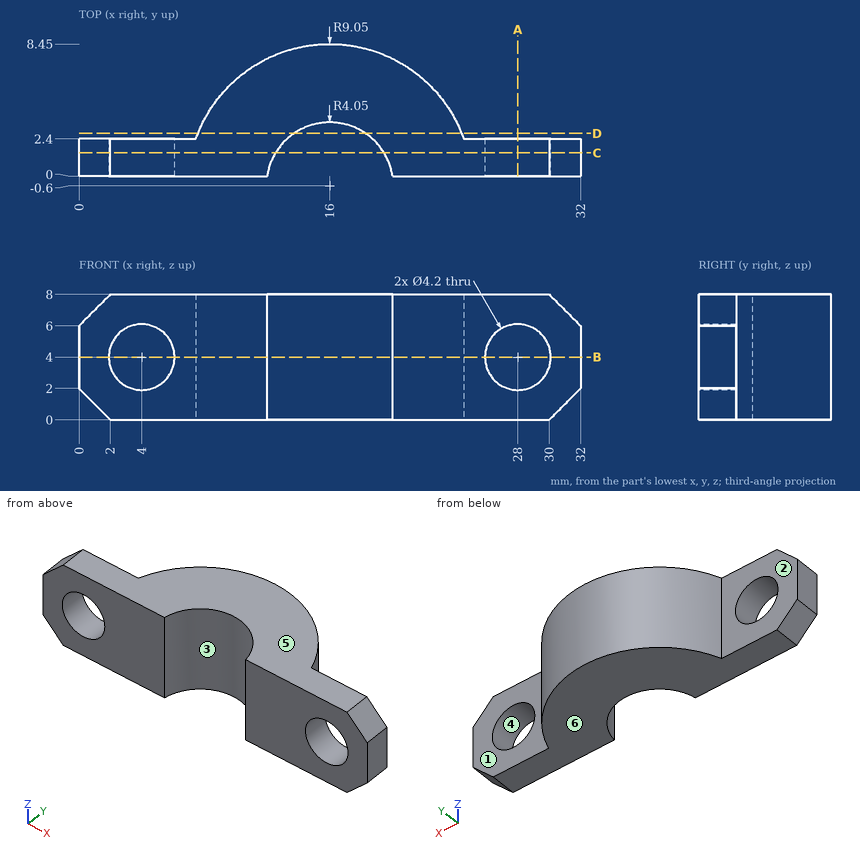
Check sheet for the drawn part. Datum: minimum x, y, z corner. Units: mm. A direction names the side the tool comes from. Coordinates: 2 decimals unless noted, no trailing zeros. Loops run counter-clockwise (first coordinate to the right, second up) from the corner with the lowest first, then second, coordinate; pieces in that order, holes last. Notation, with made-up numbers: (31, 75.25) -> (86, 75.25) arc R37 cw to (86, 114.25) -> close; hole circle Ø2 at (27, -5.75). An arc over 180 degrees is marked (long way). Write each question's results on one line, items separated by ' | '.
Item 1: Tool access check on the marked faces 1, 2 and 3. Record the directions out of +Z, -Z, +X, -X, +Y, -Y that give a thin tool (end or side, any length) a straight path to the whole face; none if there is none.
Found:
face 1: +Z, -Z, +X, +Y | face 2: +Z, -Z, -X, +Y | face 3: +Z, -Z, -Y
Item 2: Gauge pin test, flat ends, axial feed: pin 1 (1 mm diameter, centred on y = 7, z = 2, fed in from -X); pin 2 (4 mm diameter, centred on x = 18, z = 1.5, fed in from +Y); pin 3 (2 mm diameter, centred on x = 30, z = 4.5, fed in from +Y); pin 4 (1 mm diameter, centred on x = 15.5, z = 2, fed in from -Y). Record the tip position at first contact, or that the pin passes through.
Found:
pin 1: stops at x = 10.39 | pin 2: stops at y = 8.45 | pin 3: stops at y = 2.4 | pin 4: stops at y = 3.32
Item 3: Section check B-B, the plane z = 4. Enter the section's corners in (x, y), plus the area to 3 significant figures.
Found:
outline: (0, 0) -> (1.9, 0) -> (1.9, 2.4) -> (0, 2.4) -> close; (6.1, 0) -> (11.99, 0) arc R4.05 cw to (20.01, 0) -> (25.9, 0) -> (25.9, 2.4) -> (24.54, 2.4) arc R9.05 ccw to (7.46, 2.4) -> (6.1, 2.4) -> close; (30.1, 0) -> (32, 0) -> (32, 2.4) -> (30.1, 2.4) -> close | area: 111 mm2
Item 4: Material ranges on L1, parallel to Z at x = 28, y = 0.9; L2, parallel to X at y = 1.5, z = 4.5; L3, parallel to X at y = 1.75, z = 0.75, recorded low to high.
Found:
L1: z = 0 to 1.9, 6.1 to 8 | L2: x = 0 to 1.96, 6.04 to 12.54, 19.46 to 25.96, 30.04 to 32 | L3: x = 1.25 to 12.7, 19.3 to 30.75
Item 5: Mould release check, pull along Z, two halves, no side actions. Record for the marked faces 4, 5 and 6: +Z half, -Z half, draft (parallel to the pull), parting line (faces both ways), or undercut.
Found:
face 4: undercut | face 5: +Z half | face 6: -Z half
Item 6: Section check C-C, the plane y = 1.5. Enter the section's corners in (x, z).
Found:
outline: (0, 2) -> (2, 0) -> (12.54, 0) -> (12.54, 8) -> (2, 8) -> (0, 6) -> close; (19.46, 0) -> (30, 0) -> (32, 2) -> (32, 6) -> (30, 8) -> (19.46, 8) -> close; hole circle Ø4.2 at (4, 4); hole circle Ø4.2 at (28, 4)
Item 7: Section check A-A, the plane x = 28. Enter the section's corners in (y, z).
Found:
outline: (0, 0) -> (2.4, 0) -> (2.4, 1.9) -> (0, 1.9) -> close; (0, 6.1) -> (2.4, 6.1) -> (2.4, 8) -> (0, 8) -> close
Item 8: Section check D-D, the plane y = 2.75. Enter the section's corners in (x, z), plus the area to 3 significant figures.
Found:
outline: (7.59, 0) -> (13.72, 0) -> (13.72, 8) -> (7.59, 8) -> close; (18.28, 0) -> (24.41, 0) -> (24.41, 8) -> (18.28, 8) -> close | area: 98.1 mm2
